Input: dimensioned drawing with shaded views. Units: mm. Origin: part minimum x, y, z. Give positions to 0.01 mm unless a question says otherwise; leave off trailing zeros. Write each loop counter-clockwise with the first axis right and the second up, starting at its lowest first coordinate (ties: lowest second). Pieces come first, ordered by that corner, then holes.
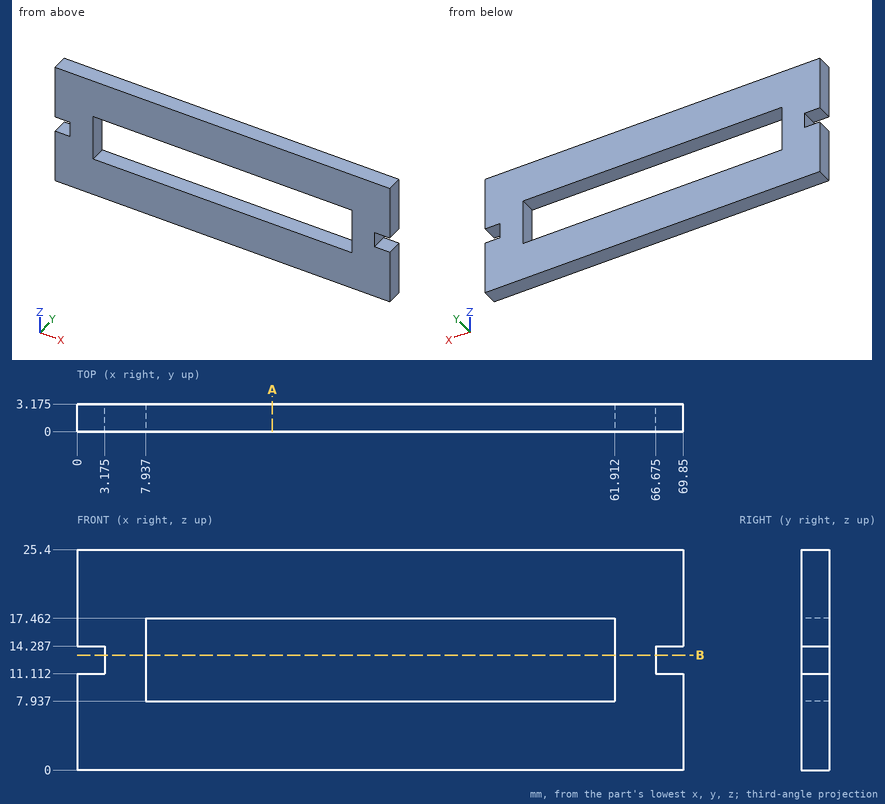
Item 1: Line query: L1, parallel to X at y = 1, z = 14.25 (1 decimal); L2, parallel to Z at x = 48.5, y = 2.55; L3, parallel to X at y = 2.6, z = 17.25. Output: solid intervals per line, ascending.
Found:
L1: x = 3.2 to 7.9, 61.9 to 66.7
L2: z = 0 to 7.94, 17.46 to 25.4
L3: x = 0 to 7.94, 61.91 to 69.85
Item 2: Section A-A, the plane x = 22.5. Return the cut outline in (y, z) (1 decimal).
Found:
outline: (0, 0) - (3.2, 0) - (3.2, 7.9) - (0, 7.9) - close; (0, 17.5) - (3.2, 17.5) - (3.2, 25.4) - (0, 25.4) - close
Item 3: Pin query (flat end, axial travel): pin 1 Ø1.5 at (x, y) = (38, 2) entering from -Z; pin 2 Ø1 at (y, z) = (1, 12) entering from +X (1 decimal). Return the tip coordinate at first contact, or that it passes through.
Found:
pin 1: stops at z = 0
pin 2: stops at x = 66.7
Item 4: Section B-B, the plane z = 13.25. Return the cut outline in (x, y) (1 decimal).
Found:
outline: (3.2, 0) - (7.9, 0) - (7.9, 3.2) - (3.2, 3.2) - close; (61.9, 0) - (66.7, 0) - (66.7, 3.2) - (61.9, 3.2) - close
